Geometry: final body of the model. Coordinates: model frame, mm. A direction names the side the tool comes from. Give positions to 0.01 mm unless a question says otherwise; leave off trailing zeros. Loops run counter-clockwise (first coordinate to the right, second up) from the corner with the lowest first, then second, coordinate; pieces in that order, holes last. Notation, with made-up numbers: (-32.75, 54) -> (-16.75, 54) arc R12 ccw to (-16.75, 62) -> close; hole circle Ø3 at (57.5, 27). An arc over 180 degrees is marked (long way). Answer in a Markdown table with one row per item. Add a question column.
1) Access query for faces 4 (the flat face through (5, 8, 22)), 5 (the flat face through (5, 8, -23)), 6 (the flat face through (5, 0, 0)). Directions: +Z, -Z, +X, -X, +Y, -Y. A direction counts if a zero-diameter tool reaches every point of the face in a straight line with its end or side. Return the directions, or none.
2) Section query D-D (y = 10). Return the cut outline in (x, z), plus the area to 3 significant figures.
3) First-contact query: P1, Ø1, axis at x = 7, z = 2, coming from the +Y side; P2, Ø2.5, axis at x = 6, z = 23.5, coming from the +Y side; P3, Ø3, axis at x = 2, z = -8.5, coming from the +Y side. Flat tips, straight axial feed; report the tip coordinate or a pass-through.
4) Draft query along Z for faces 1 (the cylindrical face through (4.93, 20.48, 0.33)), 2 (the flat face through (10, 8, 0)), 3 (the cylindrical face through (5.07, 10.85, 13.01)). Return one class per face: +Z half, -Z half, draft (parallel to the pull), parting line (faces both ways), or undercut.
5) Section query A-A (z = 0). Return the cut outline in (x, y), plus the area to 3 significant figures.
6) Section query C-C (z = -16). Return the cut outline in (x, y).
7) Line query: line 1 (Y direction, x = 8.5, z = -14); line 2 (Y direction, x = 4, z = 0); line 3 (Y direction, x = 5.75, z = -21). Output: solid intervals per line, ascending. Write a range as from..to.
```python
from build123d import *

# Parameters (mm, degrees)
SKETCH_1_R      = 2.5
EXTRUDE_1_DEPTH = 10
FILLET_1_R      = 10


with BuildPart() as part:
    # 草圖1 → 填料-伸長1 (new body)
    with BuildSketch(Plane(origin=(0, 0, 0), x_dir=(0, 0, -1), z_dir=(1, 0, 0))):
        with BuildLine():
            Line((-25, 0), (25, 0))
            Line((25, 0), (25, 8))
            Line((25, 8), (10, 8))
            Line((10, 8), (10, 18))
            ThreePointArc((10, 18), (0, 28), (-10, 18))
            Line((-10, 18), (-10, 8))
            Line((-10, 8), (-25, 8))
            Line((-25, 8), (-25, 0))
        make_face()
        with Locations((0, 18)):
            Circle(SKETCH_1_R, mode=Mode.SUBTRACT)
    extrude(amount=EXTRUDE_1_DEPTH)

    # 圓角1
    fillet_1_edges = [part.edges().sort_by_distance(p)[0] for p in [
        (5, 8, -10),
        (5, 8, 10),
    ]]
    fillet(fillet_1_edges, radius=FILLET_1_R - 0.0001)  # a hair under: the kernel refuses the full size


solid = part.part
```
Evaluation:
| question | item | result |
|---|---|---|
| 1 | face 4 | +Z, +X, -X, +Y |
| 1 | face 5 | -Z, +X, -X, +Y |
| 1 | face 6 | +Z, -Z, +X, -X, -Y |
| 2 | outline | (0, -14) -> (10, -14) -> (10, 14) -> (0, 14) -> close |
| 2 | area | 280 mm² |
| 3 | P1 | y = 27.89 |
| 3 | P2 | y = 8 |
| 3 | P3 | y = 25.14 |
| 4 | face 1 | undercut |
| 4 | face 2 | draft |
| 4 | face 3 | +Z half |
| 5 | outline | (0, 0) -> (10, 0) -> (10, 15.5) -> (0, 15.5) -> close; (0, 20.5) -> (10, 20.5) -> (10, 28) -> (0, 28) -> close |
| 5 | area | 230 mm² |
| 6 | outline | (0, 0) -> (10, 0) -> (10, 8.83) -> (0, 8.83) -> close |
| 7 | line 1 | 0..10 |
| 7 | line 2 | 0..15.5, 20.5..28 |
| 7 | line 3 | 0..8 |
